from build123d import *

# Parameters (mm, degrees)
BOSS_EXTRUDE1_DEPTH = 5.842
FILLET1_R           = 1.5875


with BuildPart() as part:
    # Sketch1 → Boss-Extrude1 (new body)
    with BuildSketch(Plane.XY):
        Polygon((12.7, -9.525), (-12.7, -9.525), (-12.7, -6.35), (-18.442, -6.35), (-18.442, -9.525), (-24.792, -9.525), (-24.792, 3.175), (-18.442, 3.175), (-12.7, 3.175), (-12.7, 9.525), (12.7, 9.525), (12.7, 3.175), (18.442, 3.175), (24.792, 3.175), (24.792, -9.525), (18.442, -9.525), (18.442, -6.35), (12.7, -6.35), align=None)
    extrude(amount=BOSS_EXTRUDE1_DEPTH)

    # Fillet1
    fillet1_edges = [part.edges().sort_by_distance(p)[0] for p in [
        (24.792, 3.175, 2.921),
        (24.792, -9.525, 2.921),
        (-24.792, -9.525, 2.921),
        (-24.792, 3.175, 2.921),
    ]]
    fillet(fillet1_edges, radius=FILLET1_R)


solid = part.part
Here's how the part is built. I have some questions about the finished solid (model axes, mm). A direction names the side the tool comes from. Round coordinates to 2 decimals unless told otherwise and drop trailing zeros. Write each loop counter-clockwise with the first axis right and the second up, starting at its lowest first coordinate (ties: lowest second). Pieces come first, ordered by that corner, then holes. Notation, with made-up numbers: (-22, 68.5) -> (-8, 68.5) arc R11 cw to (-8, 84.5) -> close; hole circle Ø9 at (57, -23). An arc over 180 degrees is marked (long way). One line per item, written item: value.
1) Suppose I cut it at C-C on x = 17. List the corners of the cut face in (y, z) for me (3 decimals), plus the area to 3 significant figures.
Filled sheet:
outline: (-6.35, 0) -> (3.175, 0) -> (3.175, 5.842) -> (-6.35, 5.842) -> close
area: 55.6 mm2
2) Suppose I cut it at B-B on y = 4.25. List the corners of the cut face in (x, z) for me.
Filled sheet:
outline: (-12.7, 0) -> (12.7, 0) -> (12.7, 5.84) -> (-12.7, 5.84) -> close
3) We'd pull the mould along X, two halves only. Please class faces 1 (the face through (-24.792, -3, 3)), 2 (the face through (0, 0, 0)), 3 (the face through (-12.7, -8, 3)): released by +X, released by -X, zero draft, split by the parting line, or undercut.
Filled sheet:
face 1: released by -X
face 2: zero draft
face 3: undercut
4) If I drill on line 1 (X direction, y = -7.5, z = 3.2); line 2 (X direction, y = 7.75, z = 0.85); line 3 (Y direction, x = 22, z = 2.25) (3 decimals), over which ranges is the centre line in solid material (lowest first)? Write a range as [from, to].
Filled sheet:
line 1: x = [-24.79, -18.44], [-12.7, 12.7], [18.44, 24.79]
line 2: x = [-12.7, 12.7]
line 3: y = [-9.525, 3.175]
5) I'm going to push flat-ended pins straight in: pin 1 Ø3 at (x, z) = (16.5, 2.5) entering from +Y (3 decimals); pin 2 Ø3 at (y, z) = (5, 3) entering from -X; pin 3 Ø1.7 at (x, z) = (-16, 2) entering from -Y; pin 4 Ø3 at (x, y) = (15.5, 7.5) entering from -Z. Where does each tip first touch, or does it pass through?
Filled sheet:
pin 1: stops at y = 3.175
pin 2: stops at x = -12.7
pin 3: stops at y = -6.35
pin 4: passes through
6) For faces 4 (the face through (0, 9.525, 3)), 5 (the face through (-18, 3.175, 3)), 6 (the face through (12.7, 6, 3)), 7 (the face through (18.442, -8, 3)), which set-ups out of +Z, -Z, +X, -X, +Y, -Y let a thin tool reach every point of the face, with its end or its side?
Filled sheet:
face 4: +Z, -Z, +X, -X, +Y
face 5: +Z, -Z, -X, +Y
face 6: +Z, -Z, +X, +Y
face 7: +Z, -Z, -Y
